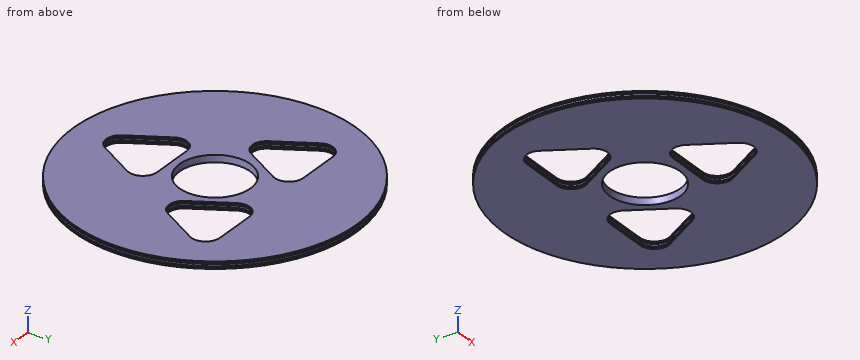
```python
from build123d import *

# Parameters (mm, degrees)
SKETCH_1_R          = 199.1381229
EXTRUDE_1_DEPTH     = 10
SKETCH_2_R          = 50
CUT_EXTRUDE_1_DEPTH = 10
SKETCH_4_W          = 2.080900767
SKETCH_4_H          = 145.70816296


with BuildPart() as part:
    # Эскиз1 → Бобышка-Вытянуть1 (new body)
    with BuildSketch(Plane.XY):
        Circle(SKETCH_1_R)
    extrude(amount=EXTRUDE_1_DEPTH)

    # Эскиз2 → Вырез-Вытянуть1 (cut)
    with BuildSketch(Plane(origin=(0, 0, 0), x_dir=(-1, 0, 0), z_dir=(0, 0, -1))):
        Circle(SKETCH_2_R)
        with BuildLine():
            Line((-132.460540699, 56.403298942), (-102.076076874, 3.945846105))
            ThreePointArc((-102.076076874, 3.945846105), (-84.74156592, -6.029860886), (-67.435094768, 3.994412468))
            Line((-67.435094768, 3.994412468), (-37.197839906, 56.536856438))
            ThreePointArc((-37.197839906, 56.536856438), (-37.225879708, 76.536836783), (-54.560390663, 86.512543774))
            Line((-54.560390663, 86.512543774), (-115.182109349, 86.427552639))
            ThreePointArc((-115.182109349, 86.427552639), (-132.488580502, 76.403279286), (-132.460540699, 56.403298942))
        make_face()
        with BuildLine():
            Line((17.383580609, -142.915842715), (47.620835471, -90.373398744))
            ThreePointArc((47.620835471, -90.373398744), (47.592795668, -70.3734184), (30.258284714, -60.397711409))
            Line((30.258284714, -60.397711409), (-30.363433973, -60.482702544))
            ThreePointArc((-30.363433973, -60.482702544), (-47.669905125, -70.506975897), (-47.641865322, -90.506956241))
            Line((-47.641865322, -90.506956241), (-17.257401498, -142.964409078))
            ThreePointArc((-17.257401498, -142.964409078), (0.077109457, -152.940116069), (17.383580609, -142.915842715))
        make_face()
        with BuildLine():
            Line((115.07696009, 86.512543774), (54.455241404, 86.427552639))
            ThreePointArc((54.455241404, 86.427552639), (37.148770252, 76.403279286), (37.176810054, 56.403298942))
            Line((37.176810054, 56.403298942), (67.561273879, 3.945846105))
            ThreePointArc((67.561273879, 3.945846105), (84.895784833, -6.029860886), (102.202255985, 3.994412468))
            Line((102.202255985, 3.994412468), (132.439510847, 56.536856438))
            ThreePointArc((132.439510847, 56.536856438), (132.411471045, 76.536836783), (115.07696009, 86.512543774))
        make_face()
    extrude(amount=-CUT_EXTRUDE_1_DEPTH, mode=Mode.SUBTRACT)

    # Эскиз4 → Вырез-Повернуть1 (revolve, cut)
    with BuildSketch(Plane(origin=(0, 0, 0), x_dir=(0, 0, -1), z_dir=(1, 0, 0))):
        with Locations((-7.572959809, 126.369713558)):
            Rectangle(SKETCH_4_W, SKETCH_4_H)
        with Locations((-2.427040192, 126.369713558)):
            Rectangle(SKETCH_4_W, SKETCH_4_H)
    revolve(axis=Axis((0, 0, 0.50000655), (0, 0, 1)), mode=Mode.SUBTRACT)


solid = part.part
```
Could you check a few things on this model? Use its own coordinates, in mm. Coordinates: 2 decimals unless noted, no trailing zeros. Loops run counter-clockwise (first coordinate to the right, second up) from the corner with the lowest first, then second, coordinate; pieces in that order, holes last.
1) Imagine slicing it at B-B (x = 91). List the corners of the cut face in (y, z) for me.
Reported:
outline: (-177.13, 0) - (-5.03, 0) - (-5.03, 1.39) - (-177.13, 1.39) - close; (-177.13, 3.47) - (-5.03, 3.47) - (-5.03, 6.53) - (-177.13, 6.53) - close; (-177.13, 8.61) - (-5.03, 8.61) - (-5.03, 10) - (-177.13, 10) - close; (86.46, 0) - (177.13, 0) - (177.13, 1.39) - (86.46, 1.39) - close; (86.46, 3.47) - (177.13, 3.47) - (177.13, 6.53) - (86.46, 6.53) - close; (86.46, 8.61) - (177.13, 8.61) - (177.13, 10) - (86.46, 10) - close
2) Imagine slicing it at A-A (y = -172.5). List the corners of the cut face in (x, z) for me.
Reported:
outline: (-99.5, 0) - (99.5, 0) - (99.5, 1.39) - (-99.5, 1.39) - close; (-99.5, 3.47) - (99.5, 3.47) - (99.5, 6.53) - (-99.5, 6.53) - close; (-99.5, 8.61) - (99.5, 8.61) - (99.5, 10) - (-99.5, 10) - close
3) Will these pins go through, and if not, where does the flat tip stop? pin 1 Ø2 at (y, z) = (48.5, 1.5) entering from +X; pin 2 Ø4 at (y, z) = (-43.5, 2.5) entering from +X.
Reported:
pin 1: stops at x = 193.39
pin 2: stops at x = 194.71
4) Imagine slicing it at C-C (x = -151). List the corners of the cut face in (y, z) for me.
Reported:
outline: (-129.83, 0) - (129.83, 0) - (129.83, 1.39) - (-129.83, 1.39) - close; (-129.83, 3.47) - (129.83, 3.47) - (129.83, 6.53) - (-129.83, 6.53) - close; (-129.83, 8.61) - (129.83, 8.61) - (129.83, 10) - (-129.83, 10) - close
5) Please list where these lines run through material, in increasing order: line 1 along Z through (x, y) = (67, -166.5); line 2 along Y through (x, z) = (0, 5); line 3 along Y through (x, z) = (37.5, 6).
Reported:
line 1: z = 0 to 1.39, 3.47 to 6.53, 8.61 to 10
line 2: y = -199.14 to -152.94, -60.44 to -50, 50 to 199.14
line 3: y = -195.58 to -108.02, -61.81 to -33.07, 33.07 to 56.01, 77 to 195.58
6) Imagine slicing it at D-D (y = 64). State how many separate pieces and enclosed holes the cut face has, and give its area (3 significant figures).
Reported:
separate pieces: 9
enclosed holes: 0
area: 1,030 mm2
